CAD build for the part. Positions are in the model's coordinates, mm. Face numbers are marked on the shaded views. A direction names the side the tool comes from. Round coordinates to 2 decimals unless told otherwise and drop trailing zeros. Loops run counter-clockwise (first coordinate to the right, second up) from the corner with the lowest first, then second, coordinate; pieces in that order, holes last.
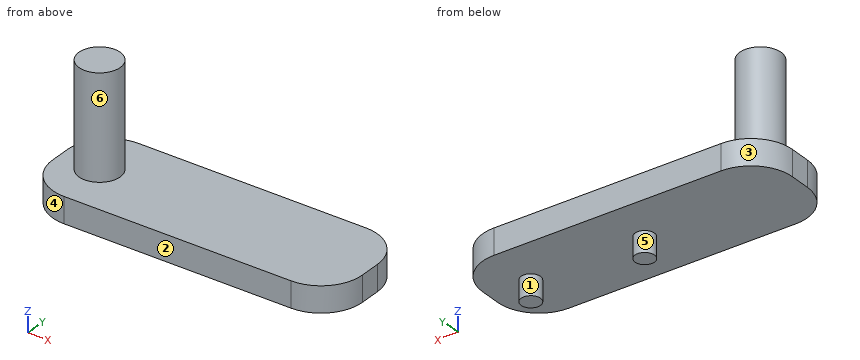
from build123d import *

# Parameters (mm, degrees)
F0_W     = 38.1
F0_H     = 3.175
F1_DEPTH = 12.7
F2_R     = 2.54
F3_DEPTH = 12.7
F4_R     = 1.1938
F5_DEPTH = 2.54
F6_R     = 1.1938
F7_DEPTH = 2.54
F8_R     = 5.08


with BuildPart() as f1:
    # F0 (on Front) → F1 (new body)
    with BuildSketch(Plane.XZ):
        with Locations((7.715251, 3.188805)):
            Rectangle(F0_W, F0_H)
    extrude(amount=F1_DEPTH)

    # F2 (on face) → F3 (join)
    with BuildSketch(Plane.XY.offset(4.776305)):
        with Locations((-6.483349, -6.35)):
            Circle(F2_R)
    extrude(amount=F3_DEPTH)

    # F4 (on face) → F5 (join)
    with BuildSketch(Plane(origin=(0, 0, 1.601305), x_dir=(1, 0, 0), z_dir=(0, 0, -1))):
        with Locations((7.410451, 5.887567)):
            Circle(F4_R)
    extrude(amount=F5_DEPTH)

    # F6 (on face) → F7 (join)
    with BuildSketch(Plane(origin=(0, 0, 1.601305), x_dir=(1, 0, 0), z_dir=(0, 0, -1))):
        with Locations((21.532176, 6.025657)):
            Circle(F6_R)
    extrude(amount=F7_DEPTH)

    # F8
    f8_edges = [f1.edges().sort_by_distance(p)[0] for p in [
        (-11.334749, -12.7, 3.188805),
        (-11.334749, 0, 3.188805),
        (26.765251, -12.7, 3.188805),
        (26.765251, 0, 3.188805),
    ]]
    fillet(f8_edges, radius=F8_R)


solid = f1.part
Item 1: Mould opens along X. For the marked faces 1, 2 and 3 say: released by +X, released by -X, zero draft, split by the parting line, or undercut.
Verdict:
face 1: undercut
face 2: zero draft
face 3: released by -X
Item 2: Wall check: L1, parallel to Z at x = 18, y = -0.75; L2, parallel to Z at x = 8, y = -5.5; L3, parallel to Y at x = -7.5, z = 8.5. Give the ranges that are in metal, low to high.
Verdict:
L1: z = 1.6 to 4.78
L2: z = -0.94 to 4.78
L3: y = -8.68 to -4.02
Item 3: Cut at D-D (z = 9). List the corners of the cut face in (x, y).
Verdict:
outline: circle Ø5.08 at (-6.48, -6.35)
Item 4: Flat gauge pins, fed straight in: P1, Ø6.5, axis at x = 6, y = -8.5, coming from the +Z side; P2, Ø4, axis at x = -5, z = 9.5, coming from the +Y side; P3, Ø3, axis at x = -4.5, y = -8, coming from the -Z side. Where does each tip first touch, or does it go through?
Verdict:
P1: stops at z = 4.78
P2: stops at y = -3.81
P3: stops at z = 1.6
Item 5: Cut at B-B (y = -8). List the corners of the cut face in (x, z), plus the area to 3 significant figures.
Verdict:
outline: (-11.32, 1.6) - (26.75, 1.6) - (26.75, 4.78) - (-4.55, 4.78) - (-4.55, 17.48) - (-8.41, 17.48) - (-8.41, 4.78) - (-11.32, 4.78) - close
area: 170 mm2
Item 6: Cut at A-A (z = 2.75). List the corners of the cut face in (x, y), plus the area to 3 significant figures.
Verdict:
outline: (-11.33, -7.62) arc R5.08 ccw to (-6.25, -12.7) - (21.69, -12.7) arc R5.08 ccw to (26.77, -7.62) - (26.77, -5.08) arc R5.08 ccw to (21.69, 0) - (-6.25, 0) arc R5.08 ccw to (-11.33, -5.08) - close
area: 462 mm2
Item 7: 3-axis set-ups, long thin cutter, end or side, ignore diameter. For the marked faces 4, 5 and 6: which of +Z, -Z, +X, -X, +Y, -Y reach the whole face in a straight line?
Verdict:
face 4: +Z, -Z, -X, -Y
face 5: -Z
face 6: +Z
Item 8: Cut at C-C (x = 19). List the corners of the cut face in (y, z).
Verdict:
outline: (-12.7, 1.6) - (0, 1.6) - (0, 4.78) - (-12.7, 4.78) - close
